Check sheet for the modelled part. Datum: model origin and axes. Units: mm. A direction names the side the tool comes from. Give positions to 0.01 mm unless a question says otherwise; leave off trailing zeros. Loops run counter-clockwise (first coordinate to the right, second up) from the corner with the lowest first, then second, coordinate; pieces in that order, holes last. Notation, with made-up numbers: M 19,-2.5 L 36,-2.5 A28 ccw 36,35.5 Z; hole C 73,12.25 d9. An arc over 180 degrees is marked long. Use one line per item in the form item = value.
from build123d import *

# Parameters (mm, degrees)
F0_W     = 762
F0_H     = 558.8
F2_DEPTH = 19.05
F3_DEPTH = 25.4
F4_DEPTH = 9.525
F5_DEPTH = 9.525
F6_DEPTH = 9.525
F7_DEPTH = 3.175
F8_R     = 6.35
F9_R     = 6.35


with BuildPart() as f2:
    # F0 (on Top) → F2 (new body)
    with BuildSketch(Plane.XY):
        with Locations((-49.2125, -76.2)):
            Rectangle(F0_W, F0_H)
    extrude(amount=-F2_DEPTH)

    # F1 (on face) → F3 (cut)
    with BuildSketch(Plane.XY):
        Polygon((-115.8875, -98.425), (-114.436071, -104.775), (-90.4875, -209.55), (17.4625, -209.55), (41.411071, -104.775), (42.8625, -98.425), (62.403797, -98.425), (138.1125, -98.425), (138.1125, 6.35), (-169.8625, 6.35), (-169.8625, -98.425), (-135.428797, -98.425), align=None)
    extrude(amount=-F3_DEPTH, mode=Mode.SUBTRACT)

    # F1 (on face) → F4 (cut)
    with BuildSketch(Plane.XY):
        Polygon((-188.9125, 25.4), (-188.9125, -104.775), (-133.977369, -104.775), (-135.428797, -98.425), (-169.8625, -98.425), (-169.8625, 6.35), (138.1125, 6.35), (138.1125, -98.425), (62.403797, -98.425), (60.952369, -104.775), (153.9875, -104.775), (153.9875, 25.4), align=None)
    extrude(amount=-F4_DEPTH, mode=Mode.SUBTRACT)

    # F1 (on face) → F5 (cut)
    with BuildSketch(Plane.XY):
        Polygon((41.411071, -104.775), (60.952369, -104.775), (62.403797, -98.425), (42.8625, -98.425), align=None)
    extrude(amount=-F5_DEPTH, mode=Mode.SUBTRACT)

    # F1 (on face) → F6 (cut)
    with BuildSketch(Plane.XY):
        Polygon((-135.428797, -98.425), (-133.977369, -104.775), (-114.436071, -104.775), (-115.8875, -98.425), align=None)
    extrude(amount=-F6_DEPTH, mode=Mode.SUBTRACT)

    # F1 (on face) → F7 (cut)
    with BuildSketch(Plane.XY):
        Polygon((-114.436071, -104.775), (-133.977369, -104.775), (-105.674512, -228.6), (32.649512, -228.6), (60.952369, -104.775), (41.411071, -104.775), (17.4625, -209.55), (-90.4875, -209.55), align=None)
    extrude(amount=-F7_DEPTH, mode=Mode.SUBTRACT)

    # F8
    f8_edges = [f2.edges().sort_by_distance(p)[0] for p in [
        (-169.8625, 6.35, -14.2875),
        (-169.8625, -98.425, -14.2875),
        (-115.8875, -98.425, -14.2875),
        (-90.4875, -209.55, -11.1125),
        (17.4625, -209.55, -11.1125),
        (42.8625, -98.425, -14.2875),
        (138.1125, -98.425, -14.2875),
        (138.1125, 6.35, -14.2875),
    ]]
    fillet(f8_edges, radius=F8_R)

    # F9
    f9_edges = [f2.edges().sort_by_distance(p)[0] for p in [
        (-188.9125, 25.4, -4.7625),
        (153.9875, 25.4, -4.7625),
        (153.9875, -104.775, -4.7625),
        (32.649512, -228.6, -1.5875),
        (-105.674512, -228.6, -1.5875),
        (-188.9125, -104.775, -4.7625),
    ]]
    fillet(f9_edges, radius=F9_R)


solid = f2.part
1) Set-up check for faces 1 (the face through (-139, -134, -19.05)), 2 (the face through (-37, -209.55, -11)), 3 (the face through (-37, -212, -3.175)): record each of +Z, -Z, +X, -X, +Y, -Y from which the full face is reachable in a straight line by a thin tool's end or side.
Evaluation:
face_1 = -Z, +X, -X, +Y, -Y
face_2 = +Z, -Z
face_3 = +Z
2) Section check B-B (x = -65.5). Record the cut outline in (y, z) (3 decimals), then the cut area to 3 significant figures.
Evaluation:
outline = M -355.6,-19.05 L -209.55,-19.05 L -209.55,-3.175 L -228.6,-3.175 L -228.6,0 L -355.6,0 Z; M 6.35,-19.05 L 203.2,-19.05 L 203.2,0 L 25.4,0 L 25.4,-9.525 L 6.35,-9.525 Z
area = 6,290 mm^2
3) Scan lines: line 1 (Y direction, x = -84, z = -10.5); line 2 (X direction, y = -204, z = -8.5); line 3 (Y direction, x = -3.5, z = -5.5). Record each from-to range of solid material in increasing order.
Evaluation:
line_1 = -355.6 to -209.55, 6.35 to 203.2
line_2 = -430.21 to -91.76, 18.73 to 331.79
line_3 = -355.6 to -209.55, 25.4 to 203.2
